from build123d import *

# Parameters (mm, degrees)
F0_W     = 304.8
F0_H     = 228.6
F1_DEPTH = 19.05
F2_SIZE2 = 7.890758
F2_SIZE  = 19.04999


# Not quite as in the source:
# - a fillet or chamfer is up to 0.001 mm smaller than in the source, because OpenCascade refuses the exact size


with BuildPart() as f1:
    # F0 (on Top) → F1 (new body)
    with BuildSketch(Plane.XY):
        Rectangle(F0_W, F0_H)
    extrude(amount=F1_DEPTH)

    # F2 (size 19.05 and 7.8907683632 in the source; OpenCascade refuses exactly that, so slightly less here)
    f2_edges = [f1.edges().sort_by_distance(p)[0] for p in [
        (0, 114.3, 19.05),
    ]]
    f2_side = f1.faces().sort_by_distance((0, 114.3, 9.525))[0]
    chamfer(f2_edges, length=F2_SIZE, length2=F2_SIZE2, reference=f2_side)


solid = f1.part
The listing builds one solid part. Answer for the finished solid, in the listing's coordinates (mm). Give positions to 0.01 mm unless a question says otherwise; leave off trailing zeros. Write each loop counter-clockwise with the first axis right and the second up, starting at its lowest first coordinate (ties: lowest second). Pieces come first, ordered by that corner, then holes. Notation, with made-up numbers: (10.25, 41) -> (47.25, 41) arc R20 ccw to (47.25, 52) -> close; hole circle Ø2 at (34.5, -7.5). An arc over 180 degrees is marked (long way). One line per question, with ' | ' between items. Start each with the question number.
1. Section B-B (z = 12) is taken. Determine the outline of the cut face in (x, y), plus the area to 3 significant figures.
2. Find the intervals of material crossed by probe 1 along Y at (x, z) = (-122.5, 3.5); probe 2 along Y at (x, z) = (-140, 2.5), in increasing order.
3. Given pin 1 Ø3 at (x, z) = (-119, 3) entering from +Y; pin 2 Ø1.5 at (x, y) = (11.5, -90.5) entering from -Z, each flat-ended and moving along its own axis, determine where each tip first touches the part or whether it passes through.
Response values:
1) outline: (-152.4, -114.3) -> (152.4, -114.3) -> (152.4, 109.33) -> (-152.4, 109.33) -> close | area: 68,200 mm2
2) probe 1: -114.3 to 112.85 | probe 2: -114.3 to 113.26
3) pin 1: y = 113.68 | pin 2: z = 0
